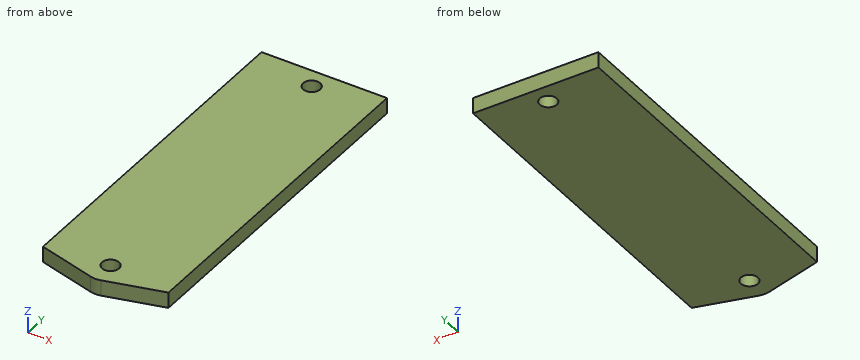
```python
from build123d import *

# Parameters (mm, degrees)
F0_R     = 1.7272
F1_DEPTH = 3.175
F2_R     = 3.96875


with BuildPart() as f1:
    # F0 (on Top) → F1 (new body)
    with BuildSketch(Plane.XY):
        Polygon((-12.7, 3.402955), (0, 0), (12.7, 3.402955), (12.7, 72.399253), (-12.7, 72.399253), align=None)
        with Locations((0, 4.930503)):
            Circle(F0_R, mode=Mode.SUBTRACT)
        with Locations((0, 68.430503)):
            Circle(F0_R, mode=Mode.SUBTRACT)
    extrude(amount=F1_DEPTH)

    # F2
    f2_edges = [f1.edges().sort_by_distance(p)[0] for p in [
        (0, 0, 1.5875),
    ]]
    fillet(f2_edges, radius=F2_R)


solid = f1.part
```
Here's how the part is built. I have some questions about the finished solid (model axes, mm). Coordinates: 2 decimals unless noted, no trailing zeros. Loops run counter-clockwise (first coordinate to the right, second up) from the corner with the lowest first, then second, coordinate; pieces in that order, holes last. Notation, with made-up numbers: (71.25, 80) - (104.25, 80) arc R8 ccw to (104.25, 93) - close; hole circle Ø4 at (-9.75, 28). An arc over 180 degrees is marked (long way). Answer as CSV lines item,"result".
Q1. If we section it at B-B, the plane z = 2.4: Write out the boundary of the cut face in (x, y).
Response:
outline,"(-12.7, 3.4) - (-1.03, 0.28) arc R3.97 ccw to (1.03, 0.28) - (12.7, 3.4) - (12.7, 72.4) - (-12.7, 72.4) - close; hole circle Ø3.45 at (0, 4.93); hole circle Ø3.45 at (0, 68.43)"
Q2. If we section it at A-A, the plane x = 0: Write out the boundary of the cut face in (y, z) (3 decimals).
Response:
outline,"(0.14, 0) - (3.203, 0) - (3.203, 3.175) - (0.14, 3.175) - close; (6.658, 0) - (66.703, 0) - (66.703, 3.175) - (6.658, 3.175) - close; (70.158, 0) - (72.399, 0) - (72.399, 3.175) - (70.158, 3.175) - close"
Q3. For pin 1 (2 mm diameter, centred on x = 7, y = 37, fed in from -Z); pin 2 (3 mm diameter, centred on x = 0, y = 4.93, fed in from -Z), each with a flat end and sliding along its axis, tell me the tip position at first contact or that it passes through.
Response:
pin 1,"z = 0"
pin 2,"through"
Q4. If I drill on L1, parallel to Y at x = 0, z = 1.5; L2, parallel to Y at x = 0.75, z = 2.7; L3, parallel to X at y = 69, z = 2.5, over which ranges is the centre line in solid material (lowest first)? Write a range as [from, to].
Response:
L1,"[0.14, 3.2], [6.66, 66.7], [70.16, 72.4]"
L2,"[0.21, 3.37], [6.49, 66.87], [69.99, 72.4]"
L3,"[-12.7, -1.63], [1.63, 12.7]"
Q5. If we section it at C-C, the plane x = 7: Write out the boundary of the cut face in (y, z) (3 decimals), and give its area (3 significant figures).
Response:
outline,"(1.876, 0) - (72.399, 0) - (72.399, 3.175) - (1.876, 3.175) - close"
area,"224 mm2"
